Study the drawing (mm; zero at the part's minimum x, y, z) and answer. Round coordinates to 2 decimals unless told otherwise and drop trailing zeros. Write each loop counter-clockwise with the first axis right and the second up, starting at its lowest first coordinate (ties: lowest second). Pieces come first, ordered by that corner, then holes. Notation, with made-up numbers: (67.5, 55.5) - (73.5, 55.5) arc R19 ccw to (73.5, 68.5) - close; hole circle Ø2 at (68, 81.25). An arc over 180 degrees is marked (long way). Return JSON: item names as keys, results as strings. Group by question number.
(1) Section A-A, the plane x = 4 is taken. Write down the section's boundary in (y, z) (1 decimal).
(2) Section B-B, the plane y = 0.9 is taken. Give the number of separate pieces and of enclosed holes in the cut face, then the cut area to 3 significant figures.
(3) Each of these flat-tipped pins is pushed along its axis until it touches: pin 1 (2 mm diameter, centred on x = 3.37, z = 3.21, fed in from -Y); pin 2 (5 mm diameter, centred on x = 31, z = 18, fed in from -Y). Where does it stop, or does it pass through?
(4) Find the intervals of material crossed by line 1 along Z through (x, y) = (10.5, 1.7); line 2 along X through (y, z) = (1.8, 34.5) (1 decimal); line 3 along X through (y, z) = (1.15, 34) (1 decimal), in increasing order. Write a range as [from, to].
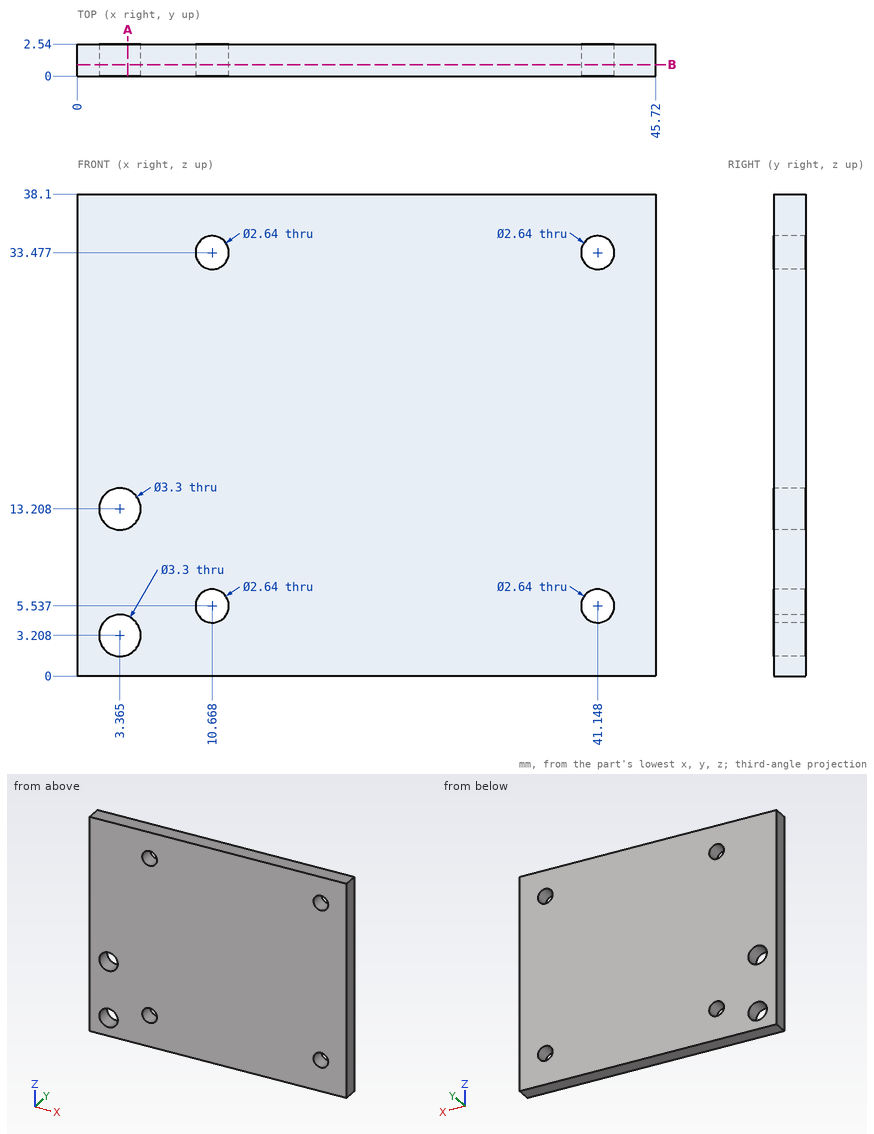
Working result:
{
 "1": {"outline": "(0, 0) - (2.5, 0) - (2.5, 1.7) - (0, 1.7) - close; (0, 4.7) - (2.5, 4.7) - (2.5, 11.7) - (0, 11.7) - close; (0, 14.7) - (2.5, 14.7) - (2.5, 38.1) - (0, 38.1) - close"},
 "2": {"separate pieces": "1", "enclosed holes": "6", "area": "1,700 mm^2"},
 "3": {"pin 1": "passes through", "pin 2": "stops at y = 0"},
 "4": {"line 1": "z = [0, 4.23], [6.85, 32.17], [34.79, 38.1]", "line 2": "x = [0, 9.8], [11.5, 40.3], [42, 45.7]", "line 3": "x = [0, 9.5], [11.9, 39.9], [42.4, 45.7]"}
}
